from build123d import *

# Parameters (mm, degrees)
EXTRUDE1_DEPTH = 28


with BuildPart() as part:
    # Sketch1 → Extrude1 (new body)
    with BuildSketch(Plane(origin=(0, 0, 0), x_dir=(1, 0, 0), z_dir=(0, 1, 0))):
        Polygon((-35.527943991, -10), (3.362928975, -48.890872965), (-44.720332146, -96.974134086), (-83.611205111, -58.083261121), align=None)
    extrude(amount=EXTRUDE1_DEPTH)

    # Sketch2 → Loft1 section 0
    with BuildSketch(Plane(origin=(0, 28, 0), x_dir=(-1, 0, 0), z_dir=(0, 1, 0)), mode=Mode.PRIVATE) as loft1_s0:
        Polygon((35.527943991, 10), (-3.362928975, 48.890872965), (44.720332146, 96.974134086), (83.611205111, 58.083261121), align=None)
    loft([Vertex(-40.124138068, 78, 53.487067043), loft1_s0.sketch])


solid = part.part
CAD build for the part. Positions are in the model's coordinates, mm. Coordinates: 2 decimals unless noted, no trailing zeros. Order: outer loops, then holes, each group sorted by start corner. A loop starts at its lowest first (then second) coordinate and runs counter-clockwise, first axis right, second up. Notation, with made-up numbers: (67, 40.5) -> (85, 40.5) arc R22 ccw to (85, 51.5) -> close; hole circle Ø11 at (27.25, 58.5). An arc over 180 degrees is marked (long way). Answer in a Markdown table with one row per item.
1) Band-saw the part on A-A (y = 8.5). List the corners of the cut face in (x, z).
Check values:
| item | result |
|---|---|
| outline | (-83.61, 58.08) -> (-35.53, 10) -> (3.36, 48.89) -> (-44.72, 96.97) -> close |
2) Band-saw the part on D-D (z = 56.5). List the corners of the cut face in (x, y).
Check values:
| item | result |
|---|---|
| outline | (-82.03, 0) -> (-4.25, 0) -> (-4.25, 28) -> (-40.44, 74.54) -> (-68.63, 45.22) -> (-82.03, 28) -> close |
3) Band-saw the part on C-C (x = -27). List the corners of the cut face in (y, z).
Check values:
| item | result |
|---|---|
| outline | (0, 18.53) -> (28, 18.53) -> (62.91, 52.1) -> (28, 79.25) -> (0, 79.25) -> close |
4) Flat gauge pins, fed straight in: P1, Ø10, axis at y = 47, z = 22, coming from the -X side; P2, Ø4, axis at x = -13.5, z = 38, coming from the +Y side; P3, Ø6, axis at x = -69, z = 37.5, coming from the -Y side; P4, Ø4, axis at y = 28.5, z = 68.5, coming from the +X side. Where does each tip first touch, or does it go through?
Check values:
| item | result |
|---|---|
| P1 | x = -39.08 |
| P2 | y = 37.15 |
| P3 | through |
| P4 | x = -14.31 |
5) Band-saw the part on B-B (z = 70). List the corners of the cut face in (x, y).
Check values:
| item | result |
|---|---|
| outline | (-71.69, 0) -> (-17.75, 0) -> (-17.75, 28) -> (-41.87, 59.01) -> (-71.69, 28) -> close |
6) Drill centre lines: line 1 (Z direction, x = -20, y = 22); line 2 (X direction, y = 44.5, z = 80); line 3 (Y direction, x = -19, z = 60). Where is each one in solid material? Low to high.
Check values:
| item | result |
|---|---|
| line 1 | 25.53 to 72.25 |
| line 2 | -45.83 to -40.58 |
| line 3 | 0 to 42.47 |
